Autodesk Inventor part; units mm, degrees
ref_plane "YZ Plane" through (0, 0, 0) normal (1, 0, 0) x (0, 1, 0)
ref_plane "XZ Plane" through (0, 0, 0) normal (0, 1, 0) x (-1, 0, 0)
ref_plane "XY Plane" through (0, 0, 0) normal (0, 0, 1) x (1, 0, 0)
sketch "Sketch1" plane through (0, 0, 0) normal (1, 0, 0) x (0, 1, 0)
  line L0 (10, 37.5) -> (10, -37.5)
  arc A0 (-10, -37.5) -> (10, -37.5) centre (0, -37.5) ccw
  line L1 (-10, -37.5) -> (-10, 37.5)
  line L2 (-10, 37.5) -> (10, 37.5)
  point P0 (0, 0)
  point P1 (-10, 0)
  dimension "d0" = 20
  dimension "d1" = 75
  dimension "d2" = 10
extrude "Extrusion1" add sketch "Sketch1" along normal mid plane 20
sketch "Sketch2" plane through (0, 0, 0) normal (1, 0, 0) x (0, 1, 0)
  line L0 (-10, 37.5) -> (10, 37.5)
  line L1 (6.1, 37.5) -> (6.1, -37.5)
  arc A0 (-6.1, -37.5) -> (6.1, -37.5) centre (0, -37.5) ccw
  line L2 (-6.1, -37.5) -> (-6.1, 37.5)
  point P0 (0, 0)
  dimension "d5" = 75
  dimension "d6" = 12.2
extrude "Extrusion2" cut sketch "Sketch2" along normal mid plane 16
fillet "Fillet1" radius 2 6 edges at (-10, 0, -47.5) (-10, 10, 0) (-10, -10, 0) (10, 0, -47.5) (10, 10, 0) (10, -10, 0)
fillet "Fillet2" radius 1 8 edges at (-9.4142, -9.4142, 37.5) (-10, 0, 37.5) (-9.4142, 9.4142, 37.5) (0, 10, 37.5) (9.4142, 9.4142, 37.5) (10, 0, 37.5) (9.4142, -9.4142, 37.5) (0, -10, 37.5)
properties part number "Part5_GOMA" material "Polystyrene"
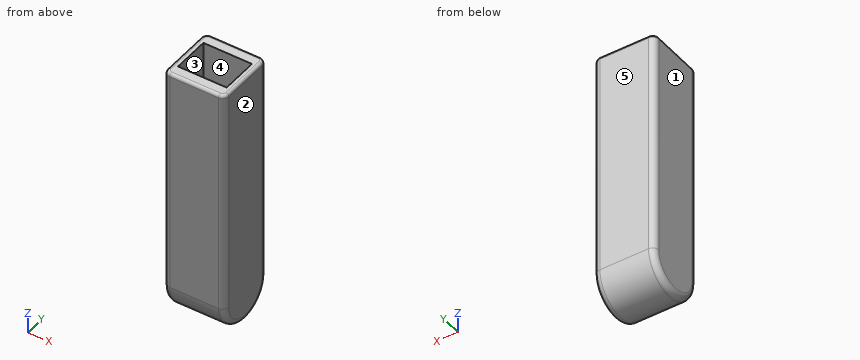
For this review, take the finished solid that the model builds, in its own axes (mm). Face numbers are marked on the shaded views. A direction names the side the tool comes from. Give positions to 0.01 mm unless a question says otherwise; leave off trailing zeros. Loops run counter-clockwise (first coordinate to the right, second up) from the corner with the lowest first, then second, coordinate; pieces in that order, holes last. Notation, with made-up numbers: (-3, 8.25) - (36, 8.25) arc R14 ccw to (36, 35.25) - close; hole circle Ø1 at (61, 72). An arc over 180 degrees is marked (long way). Write each question's results on one line, items separated by ' | '.
(1) Draft analysis for pull direction X (two halves, no side actions). For the marked faces 1, 2 and 3, state which applies: +X half, -X half, draft (parallel to the pull), parting line (faces both ways), or undercut.
Conclusion:
face 1: -X half | face 2: +X half | face 3: undercut
(2) Take a section at C-C (y = 0). Give the boundary of the cut face in (x, z), then the cut area to 3 significant figures.
Conclusion:
outline: (-10, -45.5) arc R2 ccw to (-8, -47.5) - (8, -47.5) arc R2 ccw to (10, -45.5) - (10, 36.5) arc R1 ccw to (9, 37.5) - (8, 37.5) - (8, -43.6) - (-8, -43.6) - (-8, 37.5) - (-9, 37.5) arc R1 ccw to (-10, 36.5) - close | area: 400 mm^2
(3) Take a section at A-A (z = -29). Give the boundary of the cut face in (x, y).
Conclusion:
outline: (-10, -8) arc R2 ccw to (-8, -10) - (8, -10) arc R2 ccw to (10, -8) - (10, 8) arc R2 ccw to (8, 10) - (-8, 10) arc R2 ccw to (-10, 8) - close; hole (-8, -6.1) - (8, -6.1) - (8, 6.1) - (-8, 6.1) - close
(4) For the marked faces 4 and 5, list the 3-axis set-ups (+Z, -Z, +X, -X, +Y, -Y) from which the entire face can be reached by the end or side of a thin tool; tool diameter is ignored.
Conclusion:
face 4: +Z | face 5: +Z, -Z, +X, -X, +Y
(5) Take a section at B-B (x = -2). Give the boundary of the cut face in (y, z).
Conclusion:
outline: (-10, -37.5) arc R10 ccw to (10, -37.5) - (10, 36.5) arc R1 ccw to (9, 37.5) - (6.1, 37.5) - (6.1, -37.5) arc R6.1 cw to (-6.1, -37.5) - (-6.1, 37.5) - (-9, 37.5) arc R1 ccw to (-10, 36.5) - close
(6) For pin 1 Ø5 at (x, y) = (-3, -2.5) entering from +Z; pin 2 Ø12 at (x, y) = (-5, -8) entering from -Z, all flat-tipped, find the tip position at first contact; note any pin that passes through.
Conclusion:
pin 1: z = -40.99 | pin 2: z = -47.3
(7) For line 1 along Y through (x, z) = (4, -17.5); line 2 along X through (y, z) = (-6, -7.5); line 3 along Y through (x, z) = (4, -39), list the stretches that pass through material, from the lowest coordinate up.
Conclusion:
line 1: -10 to -6.1, 6.1 to 10 | line 2: -10 to -8, 8 to 10 | line 3: -9.89 to -5.91, 5.91 to 9.89
